Design review of the part built by this model. Coordinates are the model's own, in mm. A direction names the side the tool comes from. Coordinates: 2 decimals unless noted, no trailing zeros. Loops run counter-clockwise (first coordinate to the right, second up) from the corner with the lowest first, then second, coordinate; pieces in that order, holes last. Notation, with made-up numbers: (45.25, 80.5) -> (59.25, 80.5) arc R22 cw to (59.25, 86.5) -> close; hole circle Ø2 at (-24.75, 44.25). An arc over 180 degrees is marked (long way). One line per item, written item: value. Start each with the question number.
1. Machinability: for faces 1 (the flat face through (78.1, 9.4, 20)), 2 (the flat face through (20, -45, 69)), 3 (the cylindrical face through (-44, 0, 52)), 4 (the flat face through (55, -20, 52)), which of the approach directions +Z, -Z, +X, -X, +Y, -Y give a long, thin tool a straight path to every point of the face, cutting with its end or side? Answer none if there is none.
2. Add section D-D on z = 56.5. Give the number of separate pieces and of enclosed holes in the cut face, plus the area to 3 significant figures.
3. For probe 1 along Y at (x, z) = (60, 61); probe 2 along X at (y, z) = (10, 18.5); probe 3 along Y at (x, z) = (-19, 49), list the stretches that pass through material, from the lowest coordinate up.
4. Insertion check: pin 1 (4 mm diameter, centred on x = -57.5, z = 33.5, fed in from +Y); pin 2 (1.5 mm diameter, centred on x = 25.5, z = 69.5, fed in from -Y); pin 3 (5 mm diameter, centred on y = -43, z = 74.5, fed in from +X). Each pin has a flat end and moves straight along its axis. Give the tip position at first contact, or say it passes through.
5. Add section C-C on z = 18. Write out the cut boundary in (x, y), plus the area to 3 significant figures.
6. Add section A-A on x = 0. Write out the cut boundary in (y, z), plus the area to 3 significant figures.
7. Draft analysis for pull direction X (two halves, no side actions). For faces 5 (the flat face through (-55, -20, 52)), 6 (the cylindrical face through (-44.262, -30.934, 52.045)), 7 (the cylindrical face through (0.3, -22.5, 10.1)), state which applies: pulls with the +X half, pulls with the -X half, needs draft (parallel to the pull), parting line crosses it, or undercut.
8. Add section B-B on y = 0. Write out the cut boundary in (x, z), plus the area to 3 significant figures.
```python
from build123d import *

# Parameters (mm, degrees)
EXTRUDE_1_DEPTH     = 20
EXTRUDE_2_DEPTH     = 65
SKETCH_4_R          = 7.5
CUT_EXTRUDE_1_DEPTH = 85
CUT_EXTRUDE_2_DEPTH = 20
EXTRUDE_3_DEPTH     = 10
SKETCH_7_R          = 9
CUT_EXTRUDE_3_DEPTH = 20
FILLET_1_R          = 5


with BuildPart() as part:
    # 草图1 → 凸台-拉伸1 (new body)
    with BuildSketch(Plane.XY):
        with BuildLine():
            Line((76, -40), (-76, -40))
            ThreePointArc((-76, -40), (-83.071067812, -37.071067812), (-86, -30))
            Line((-86, -30), (-86, 30))
            ThreePointArc((-86, 30), (-83.071067812, 37.071067812), (-76, 40))
            Line((-76, 40), (76, 40))
            ThreePointArc((76, 40), (83.071067812, 37.071067812), (86, 30))
            Line((86, 30), (86, -30))
            ThreePointArc((86, -30), (83.071067812, -37.071067812), (76, -40))
        make_face()
    extrude(amount=EXTRUDE_1_DEPTH)

    # 草图3 → 凸台-拉伸2 (add)
    with BuildSketch(Plane.XY.offset(20)):
        with BuildLine():
            Line((-36.276714294, 40), (36.276714294, 40))
            ThreePointArc((36.276714294, 40), (44.36006499, 30.792606809), (50.159744816, 20))
            Line((50.159744816, 20), (60, 20))
            ThreePointArc((60, 20), (80, 0), (60, -20))
            Line((60, -20), (50.159744816, -20))
            ThreePointArc((50.159744816, -20), (44.36006499, -30.792606809), (36.276714294, -40))
            Line((36.276714294, -40), (-36.276714294, -40))
            ThreePointArc((-36.276714294, -40), (-44.36006499, -30.792606809), (-50.159744816, -20))
            Line((-50.159744816, -20), (-60, -20))
            ThreePointArc((-60, -20), (-80, 0), (-60, 20))
            Line((-60, 20), (-50.159744816, 20))
            ThreePointArc((-50.159744816, 20), (-44.36006499, 30.792606809), (-36.276714294, 40))
        make_face()
        with BuildLine():
            Line((32.186953879, -30), (-32.186953879, -30))
            ThreePointArc((-32.186953879, -30), (-44, 0), (-32.186953879, 30))
            Line((-32.186953879, 30), (32.186953879, 30))
            ThreePointArc((32.186953879, 30), (44, 0), (32.186953879, -30))
        make_face(mode=Mode.SUBTRACT)
    extrude(amount=EXTRUDE_2_DEPTH)

    # 草图4 → 切除-拉伸1 (cut)
    with BuildSketch(Plane.XY.offset(85)):
        with Locations((-60, 0)):
            Circle(SKETCH_4_R)
        with Locations((60, 0)):
            Circle(SKETCH_4_R)
    extrude(amount=-CUT_EXTRUDE_1_DEPTH, mode=Mode.SUBTRACT)

    # 草图5 → 切除-拉伸2 (cut)
    with BuildSketch(Plane.XY.offset(20)):
        with BuildLine():
            Line((-18.708286934, -12.5), (-30, -12.5))
            Line((-30, -12.5), (-30, 12.5))
            Line((-30, 12.5), (-18.708286934, 12.5))
            ThreePointArc((-18.708286934, 12.5), (0, 22.5), (18.708286934, 12.5))
            Line((18.708286934, 12.5), (30, 12.5))
            Line((30, 12.5), (30, -12.5))
            Line((30, -12.5), (18.708286934, -12.5))
            ThreePointArc((18.708286934, -12.5), (0, -22.5), (-18.708286934, -12.5))
        make_face()
    extrude(amount=-CUT_EXTRUDE_2_DEPTH, mode=Mode.SUBTRACT)

    # 草图6 → 凸台-拉伸3 (add)
    with BuildSketch(Plane.XZ.offset(40)):
        with BuildLine():
            Line((20, 53), (20, 85))
            Line((20, 85), (-20, 85))
            Line((-20, 85), (-20, 53))
            ThreePointArc((-20, 53), (0, 33), (20, 53))
        make_face()
    extrude(amount=EXTRUDE_3_DEPTH)

    # 草图7 → 切除-拉伸3 (cut)
    with BuildSketch(Plane.XZ.offset(50)):
        with Locations((0, 53)):
            Circle(SKETCH_7_R)
    extrude(amount=-CUT_EXTRUDE_3_DEPTH, mode=Mode.SUBTRACT)

    # 圆角1
    fillet_1_edges = [part.edges().sort_by_distance(p)[0] for p in [
        (32.186953879, 30, 52.5),
        (-32.186953879, 30, 52.5),
        (-32.186953879, -30, 52.5),
        (32.186953879, -30, 52.5),
    ]]
    fillet(fillet_1_edges, radius=FILLET_1_R)


solid = part.part
```
Worked answers:
1. face 1: +Z, +X
1. face 2: +Z, -Z, +X, -Y
1. face 3: +Z
1. face 4: +Z, +X, -Y
2. separate pieces: 1
2. enclosed holes: 2
2. area: 4,490 mm²
3. probe 1: y = -20 to -7.5, 7.5 to 20
3. probe 2: x = -86 to -30, 30 to 86
3. probe 3: y = -50 to -30, 30 to 40
4. pin 1: stops at y = 20
4. pin 2: stops at y = -40
4. pin 3: stops at x = 20
5. outline: (-86, -30) arc R10 ccw to (-76, -40) -> (76, -40) arc R10 ccw to (86, -30) -> (86, 30) arc R10 ccw to (76, 40) -> (-76, 40) arc R10 ccw to (-86, 30) -> close; hole circle Ø15 at (-60, 0); hole (-30, -12.5) -> (-18.71, -12.5) arc R22.5 ccw to (18.71, -12.5) -> (30, -12.5) -> (30, 12.5) -> (18.71, 12.5) arc R22.5 ccw to (-18.71, 12.5) -> (-30, 12.5) -> close; hole circle Ø15 at (60, 0)
5. area: 11,300 mm²
6. outline: (-50, 33) -> (-40, 33) -> (-40, 0) -> (-22.5, 0) -> (-22.5, 20) -> (-30, 20) -> (-30, 44) -> (-50, 44) -> close; (-50, 62) -> (-30, 62) -> (-30, 85) -> (-50, 85) -> close; (22.5, 0) -> (40, 0) -> (40, 85) -> (30, 85) -> (30, 20) -> (22.5, 20) -> close
6. area: 2,160 mm²
7. face 5: needs draft
7. face 6: pulls with the -X half
7. face 7: undercut
8. outline: (-86, 0) -> (-67.5, 0) -> (-67.5, 85) -> (-80, 85) -> (-80, 20) -> (-86, 20) -> close; (-52.5, 0) -> (-30, 0) -> (-30, 20) -> (-44, 20) -> (-44, 85) -> (-52.5, 85) -> close; (30, 0) -> (52.5, 0) -> (52.5, 85) -> (44, 85) -> (44, 20) -> (30, 20) -> close; (67.5, 0) -> (86, 0) -> (86, 20) -> (80, 20) -> (80, 85) -> (67.5, 85) -> close
8. area: 4,370 mm²
